Work out the finished part from the listing and answer in its coordinate system (mm). A direction names the side the tool comes from. Give positions to 0.01 mm unless a question says otherwise; leave off trailing zeros. Write each loop counter-clockwise with the first axis right and the second up, starting at its lowest first coordinate (ties: lowest second). Pieces come first, ordered by that corner, then holes. Notation, with made-up numbers: (48.5, 51) - (83.5, 51) arc R29 ccw to (83.5, 89) - close; hole circle Ø2 at (-26.75, 83). An arc over 180 degrees is marked (long way). Write each question's results on one line, items separated by ' | '. Start each with the question number.
Autodesk Inventor part; units mm, degrees
ref_plane "YZ Plane" through (0, 0, 0) normal (1, 0, 0) x (0, 1, 0)
ref_plane "XZ Plane" through (0, 0, 0) normal (0, 1, 0) x (-1, 0, 0)
ref_plane "XY Plane" through (0, 0, 0) normal (0, 0, 1) x (1, 0, 0)
sketch "Sketch1" plane through (0, 0, 0) normal (0, 0, 1) x (1, 0, 0)
  line L0 (-4, 24) -> (4, 24)
  line L1 (4, 24) -> (4, -24)
  line L2 (4, -24) -> (-4, -24)
  line L3 (-4, -24) -> (-4, 24)
  point P0 (0, 0)
  dimension "d0" = 8
  dimension "d1" = 48
  dimension "d2" = 4
  dimension "d3" = 24
extrude "Extrusion1" add sketch "Sketch1" along normal blind 3.2
shell "Shell1" thickness 1.5 removed faces 1 at (-1.3333, 8, 0)
sketch "Sketch2" plane through (0, 0, 3.2) normal (0, 0, 1) x (1, 0, 0)
  circle A0 centre (0, -20) radius 2.5
  line L0 (4, 24) -> (4, -24)
  line L1 (4, -24) -> (-4, -24)
  dimension "d7" = 5
  dimension "d10" = 4
  dimension "d11" = 4
extrude "Extrusion2" add sketch "Sketch2" along normal blind 1.6
sketch "Sketch3" plane through (2.5, -22.5, 1.7) normal (0, 0, -1) x (-1, 0, 0)
  circle A0 centre (2.5, 2.5) radius 2.5
  circle A1 centre (2.5, 2.5) radius 1.2
  point P0 (2.5, 22.5)
  dimension "d18" = 2.4
extrude "Extrusion3" cut sketch "Sketch3" against normal blind 1.6 contours A1
pattern_linear "Rectangular Pattern1" count 6 spacing 8 along (0, 1, 0) of "Extrusion2", "Extrusion3"
sketch "Sketch4" plane through (2.5, -22.5, 1.7) normal (0, 0, -1) x (-1, 0, 0)
  circle A0 centre (2.5, 10.5) radius 1.2
  circle A1 centre (2.5, 2.5) radius 1.2
  line L0 (0, 45) -> (0, 0)
  line L1 (0, 0) -> (5, 0)
  circle A2 centre (6.5, 6.5) radius 3.15
  circle A3 centre (6.5, 6.5) radius 2.5
  point P0 (2.5, 22.5)
  dimension "d21" = 6.5
  dimension "d22" = 6.5
  dimension "d23" = 10.5
  dimension "d24" = 2.5
  dimension "d25" = 5
  dimension "d26" = 6.3
extrude "Extrusion4" [suppressed]
pattern_linear "Rectangular Pattern2" [suppressed]
equation "\"d0\" = 0.8 * WIDTH"
equation "\"d1\" = 0.8 * LENGTH"
equation "\"d4\" = HEIGHT"
equation "\"d21\" = 0.5 * d23 + 0.5 * d24"
equation "\"d22\" = d21"
equation "\"WIDTH\" = 1"
equation "\"HEIGHT\" = 3.2"
properties part number "3666" material "Steel"
Q1. Given pin 1 (1.2 mm diameter, centred on x = 0, y = -12, fed in from -Z); pin 2 (1.9 mm diameter, centred on x = 0.5, y = 20, fed in from -Z); pin 3 (4 mm diameter, centred on x = -1, y = 9, fed in from -Z), each flat-ended and moving along its own axis, determine where each tip first touches the part or whether it passes through.
Q2. A tool of negligible diameter and unlimited length cuts with its end or side. For faces 5 (the flat face through (-2.5, 0, 1)), 6 (the flat face through (-3, 0, 0)), 7 (the cylindrical face through (-0.33, -6.48, 3.99)), from which of +Z, -Z, +X, -X, +Y, -Y can it reach the whole face along a straight path? Write none if from no direction.
Q3. A cutting plane is placed at A-A, the plane z = 0.75. Write down the section's boundary in (x, y), and give its area (3 significant figures).
Q4. A cutting plane is placed at D-D, the plane y = 4.5. Write down the section's boundary in (x, z).
Q5. The mould has two halves that part along X. Classify faces 1 (the flat face through (4, 0, 2)), 2 (the flat face through (0, -20, 3.3)), 3 (the cylindrical face through (0.26, 18.83, 2.49)), 4 (the flat face through (0, 24, 2)): pulls with the +X half, pulls with the -X half, needs draft (parallel to the pull), parting line crosses it, or undercut.
Q6. A cutting plane is placed at C-C, the plane y = 14. Write down the section's boundary in (x, z), and give its area (3 significant figures).
Q7. A cutting plane is placed at B-B, the plane y = -4. Write down the section's boundary in (x, z), and give its area (3 significant figures).
Q8. Consider L1, parallel to X at y = -19.5, z = 1.55; L2, parallel to X at y = -10, z = 4.3; L3, parallel to Z at x = 1.5, y = -19. Determine where each line is inside the solid, lowest interval first.
Result:
1) pin 1: stops at z = 3.3 | pin 2: stops at z = 1.7 | pin 3: stops at z = 0
2) face 5: -Z | face 6: -Z, +X, -X, +Y, -Y | face 7: +Z
3) outline: (-4, -24) - (4, -24) - (4, 24) - (-4, 24) - close; hole (-2.5, -22.5) - (2.5, -22.5) - (2.5, 22.5) - (-2.5, 22.5) - close | area: 159 mm2
4) outline: (-4, 0) - (-2.5, 0) - (-2.5, 1.7) - (-1.09, 1.7) - (-1.09, 3.3) - (1.09, 3.3) - (1.09, 1.7) - (2.5, 1.7) - (2.5, 0) - (4, 0) - (4, 3.2) - (2.45, 3.2) - (2.45, 4.8) - (-2.45, 4.8) - (-2.45, 3.2) - (-4, 3.2) - close
5) face 1: pulls with the +X half | face 2: undercut | face 3: undercut | face 4: needs draft
6) outline: (-4, 0) - (-2.5, 0) - (-2.5, 1.7) - (2.5, 1.7) - (2.5, 0) - (4, 0) - (4, 3.2) - (1.5, 3.2) - (1.5, 4.8) - (-1.5, 4.8) - (-1.5, 3.2) - (-4, 3.2) - close | area: 21.9 mm2
7) outline: (-4, 0) - (-2.5, 0) - (-2.5, 1.7) - (-1.2, 1.7) - (-1.2, 3.3) - (1.2, 3.3) - (1.2, 1.7) - (2.5, 1.7) - (2.5, 0) - (4, 0) - (4, 3.2) - (2.5, 3.2) - (2.5, 4.8) - (-2.5, 4.8) - (-2.5, 3.2) - (-4, 3.2) - close | area: 21.3 mm2
8) L1: x = -4 to -2.5, 2.5 to 4 | L2: x = -1.5 to 1.5 | L3: z = 1.7 to 4.8
